```python
from build123d import *

# Parameters (mm, degrees)
SKETCH1_W               = 8
SKETCH1_H               = 8
BOSS_EXTRUDE1_DEPTH     = 3
CUT_EXTRUDE1_DEPTH      = 12.704699911
CUT_EXTRUDE1_DEPTH_BACK = 12.704699911
CUT_EXTRUDE2_DEPTH      = 11
SKETCH4_R               = 1.75
CUT_EXTRUDE3_DEPTH      = 0.4
SKETCH5_W               = 8
SKETCH5_H               = 1
BOSS_EXTRUDE2_DEPTH     = 2
FILLET1_R               = 4
CUT_EXTRUDE4_DEPTH      = 0.4
CUT_EXTRUDE5_DEPTH      = 0.5


with BuildPart() as part:
    # Sketch1 → Boss-Extrude1 (new body)
    with BuildSketch(Plane(origin=(0, 0, 0), x_dir=(1, 0, 0), z_dir=(0, 1, 0))):
        with Locations((4, 4)):
            Rectangle(SKETCH1_W, SKETCH1_H)
    extrude(amount=BOSS_EXTRUDE1_DEPTH)

    # Sketch2 → Cut-Extrude1 (cut, two sides: drawn at the far end of the back side and taken through both)
    with BuildSketch(Plane.XY.offset(-CUT_EXTRUDE1_DEPTH_BACK)):
        Polygon((0, 0), (0.6, 3), (0, 3), align=None)
        Polygon((8, 0), (7.4, 3), (8, 3), align=None)
    extrude(amount=CUT_EXTRUDE1_DEPTH + CUT_EXTRUDE1_DEPTH_BACK, mode=Mode.SUBTRACT)

    # Sketch3 → Cut-Extrude2 (cut)
    with BuildSketch(Plane(origin=(0, 0, 0), x_dir=(0, 0, -1), z_dir=(1, 0, 0))):
        Polygon((0, 0), (0.6, 3), (0, 3), align=None)
        Polygon((8, 3), (7.4, 3), (8, 0), align=None)
    extrude(amount=CUT_EXTRUDE2_DEPTH, mode=Mode.SUBTRACT)

    # Sketch4 → Cut-Extrude3 (cut)
    with BuildSketch(Plane.XZ):
        with Locations(Location((4, -3.75, 0), (0, 0, 270))):
            Circle(SKETCH4_R)
    extrude(amount=-CUT_EXTRUDE3_DEPTH, mode=Mode.SUBTRACT)

    # Sketch5 → Boss-Extrude2 (add)
    with BuildSketch(Plane.XZ):
        with Locations((4, -7.5)):
            Rectangle(SKETCH5_W, SKETCH5_H)
    extrude(amount=BOSS_EXTRUDE2_DEPTH)

    # Fillet1
    # the kernel refuses this fillet: 4 mm, written as the material it takes off along each edge
    with BuildSketch(Plane(origin=(8, -2, -16.660254038), x_dir=(0, 1, 0), z_dir=(0, 0, 1)), Plane(origin=(0, -2, 1.660254038), x_dir=(0, 1, 0), z_dir=(0, 0, -1))) as fillet1_piece_1:
        with BuildLine():
            CenterArc((4, 3.464101615), FILLET1_R, 180, 60)
            Line((0, 3.464101615), (-0.08, 3.464101615))
            Line((-0.08, 3.464101615), (-0.08, 0))
            Line((-0.08, 0), (0, -0.08))
            ThreePointArc((0, -0.08), (1, -0.08), (1.96, -0.069282032))
            Line((1.96, -0.069282032), (2, 0))
        make_face()
    extrude(amount=18.320508076, mode=Mode.SUBTRACT)

    # Sketch6 → Cut-Extrude4 (cut)
    with BuildSketch(Plane(origin=(0, 3, 0), x_dir=(1, 0, 0), z_dir=(0, 1, 0))):
        Polygon((3.623842243, 2.056832464), (3.623842243, 3.740326053), (2.162303782, 6.056832464), (3.062143525, 6.056832464), (4.007656346, 4.408595284), (4.95477173, 6.056832464), (5.854611474, 6.056832464), (4.393073013, 3.734717079), (4.393073013, 2.056832464), align=None)
    extrude(amount=-CUT_EXTRUDE4_DEPTH, mode=Mode.SUBTRACT)

    # Sketch7 → Cut-Extrude5 (cut)
    with BuildSketch(Plane(origin=(0, 3, 0), x_dir=(1, 0, 0), z_dir=(0, 1, 0))):
        with BuildLine():
            Line((6.99657775, 2.307478491), (6.650423904, 2.269617914))
            add(Edge.make_bspline(
                [(6.650423904, 2.269617914), (6.648104786, 2.286290214), (6.643740629, 2.317664439), (6.630814222, 2.360960848), (6.6128192, 2.397384178), (6.589720846, 2.426985356), (6.562208273, 2.449767653), (6.53085918, 2.465955864), (6.495693494, 2.475565581), (6.471038508, 2.476713937), (6.458236404, 2.477310221)],
                knots=[0, 0, 0, 0, 1.280716388, 2.410074291, 3.425374506, 4.35753932, 5.248331359, 6.12451615, 7.026154803, 8, 8, 8, 8], degree=3))
            add(Edge.make_bspline(
                [(6.458236404, 2.477310221), (6.449554942, 2.477097941), (6.432279271, 2.476675513), (6.407115159, 2.471312362), (6.382853927, 2.463353411), (6.359693582, 2.452081234), (6.337518567, 2.437536581), (6.316665994, 2.419545601), (6.296177185, 2.39905664), (6.277258092, 2.37431526), (6.259107425, 2.34501973), (6.243478966, 2.309156475), (6.229549311, 2.266758815), (6.217622545, 2.217619097), (6.206799126, 2.162049229), (6.197926997, 2.099824257), (6.190827571, 2.030888275), (6.1874217, 1.982610246), (6.18564025, 1.957358298)],
                knots=[0, 0, 0, 0, 0.642458078, 1.278459126, 1.898279436, 2.531842133, 3.181731979, 3.858193002, 4.57010051, 5.325711302, 6.161524323, 7.118599443, 8.217371811, 9.466325973, 10.864147948, 12.412648259, 14.123626419, 16, 16, 16, 16], degree=3))
            add(Edge.make_bspline(
                [(6.18564025, 1.957358298), (6.196703374, 1.969374309), (6.218396997, 1.992936442), (6.254393564, 2.023656049), (6.292105324, 2.049919261), (6.331942634, 2.071465901), (6.374122941, 2.087500286), (6.417882183, 2.099674887), (6.463793169, 2.1064945), (6.494994081, 2.107544715), (6.510880634, 2.108079452)],
                knots=[0, 0, 0, 0, 1.057745406, 2.074127497, 3.059409796, 4.031705469, 5.000875988, 5.977809597, 6.970362319, 8, 8, 8, 8], degree=3))
            add(Edge.make_bspline(
                [(6.510880634, 2.108079452), (6.528809934, 2.107563089), (6.564213931, 2.106543456), (6.616372239, 2.099391957), (6.666421561, 2.086532277), (6.714588312, 2.069136373), (6.761110551, 2.047230594), (6.805098359, 2.019501147), (6.847242227, 1.987169858), (6.886962554, 1.950231753), (6.923455982, 1.909566001), (6.95567607, 1.865643773), (6.982192143, 1.818330938), (7.00486021, 1.76868676), (7.021726117, 1.715731209), (7.033968982, 1.660226315), (7.04127711, 1.601662587), (7.042239139, 1.561706039), (7.042731596, 1.541252529)],
                knots=[0, 0, 0, 0, 0.99135015, 1.957564468, 2.903754199, 3.843479786, 4.78583385, 5.741106244, 6.712813504, 7.719198368, 8.735844933, 9.730198001, 10.724351158, 11.729813921, 12.742848014, 13.790983496, 14.86921809, 16, 16, 16, 16], degree=3))
            add(Edge.make_bspline(
                [(7.042731596, 1.541252529), (7.042231952, 1.519599685), (7.041257525, 1.477371451), (7.034085066, 1.415527203), (7.021415455, 1.357153196), (7.004106031, 1.301781092), (6.981716795, 1.249849655), (6.954594052, 1.200930916), (6.921819947, 1.155860856), (6.884881845, 1.114033218), (6.84370317, 1.076707467), (6.799818397, 1.043655074), (6.752740779, 1.016179585), (6.703166183, 0.993054256), (6.650243128, 0.9760833), (6.594904638, 0.963355935), (6.536700741, 0.955593381), (6.496962304, 0.954693712), (6.476625827, 0.954233298)],
                knots=[0, 0, 0, 0, 1.13287417, 2.209376133, 3.25169942, 4.254157582, 5.240146322, 6.205890558, 7.174579019, 8.150183866, 9.1206468, 10.07783463, 11.019441811, 11.967766696, 12.934309213, 13.921380422, 14.936249089, 16, 16, 16, 16], degree=3))
            add(Edge.make_bspline(
                [(6.476625827, 0.954233298), (6.454835686, 0.954842926), (6.411992392, 0.956041562), (6.349274568, 0.965905733), (6.289647802, 0.982594351), (6.233119501, 1.005900716), (6.179219819, 1.035216515), (6.128449255, 1.071632083), (6.080942348, 1.114800151), (6.036070744, 1.164136126), (5.995238787, 1.221123075), (5.960465944, 1.286988003), (5.930975089, 1.361009558), (5.906965213, 1.443377578), (5.888431321, 1.534085529), (5.875498792, 1.633141016), (5.86690889, 1.740380226), (5.866183985, 1.814672002), (5.865808519, 1.853151567)],
                knots=[0, 0, 0, 0, 0.852151446, 1.675481364, 2.476404467, 3.269281233, 4.062617998, 4.871616733, 5.707301388, 6.56955125, 7.476395267, 8.442009786, 9.475854496, 10.58877921, 11.794095973, 13.094195288, 14.494932947, 16, 16, 16, 16], degree=3))
            add(Edge.make_bspline(
                [(5.865808519, 1.853151567), (5.866346697, 1.892590697), (5.867386586, 1.968796599), (5.875754473, 2.078827487), (5.889046125, 2.180436336), (5.908408745, 2.273394012), (5.933175033, 2.357893394), (5.963200156, 2.434104295), (5.99923844, 2.501750812), (6.041138584, 2.560612949), (6.087240817, 2.61177964), (6.136777869, 2.655945181), (6.189560624, 2.693536639), (6.245587817, 2.724459089), (6.305319384, 2.747901225), (6.368188753, 2.764829378), (6.434301522, 2.775708833), (6.479587723, 2.776770851), (6.502587365, 2.777310221)],
                knots=[0, 0, 0, 0, 1.491699013, 2.882321987, 4.171520357, 5.365488089, 6.470299549, 7.49861535, 8.458736801, 9.361983288, 10.224742848, 11.058789056, 11.867429157, 12.671146298, 13.473202851, 14.288259215, 15.130652936, 16, 16, 16, 16], degree=3))
            add(Edge.make_bspline(
                [(6.502587365, 2.777310221), (6.518832845, 2.777017956), (6.550590682, 2.776446616), (6.597136362, 2.770379458), (6.641540508, 2.76110179), (6.683919501, 2.748259344), (6.723974963, 2.731060825), (6.761865954, 2.710109046), (6.797719857, 2.685460752), (6.831350121, 2.657274635), (6.862486078, 2.625465393), (6.890601127, 2.589961055), (6.915881459, 2.551190115), (6.938437714, 2.509184749), (6.957357529, 2.46354265), (6.973622233, 2.414622738), (6.98699882, 2.362319913), (6.993336088, 2.326037695), (6.99657775, 2.307478491)],
                knots=[0, 0, 0, 0, 1.036027791, 2.025301876, 2.989435482, 3.928225244, 4.845595412, 5.765526461, 6.686607585, 7.61747015, 8.561102691, 9.521661062, 10.50224679, 11.510949117, 12.559251378, 13.650572309, 14.798212656, 16, 16, 16, 16], degree=3))
        make_face()
        with BuildLine():
            add(Edge.make_bspline(
                [(6.211962365, 1.549185221), (6.212093793, 1.537753077), (6.212350595, 1.515415322), (6.216561681, 1.483001611), (6.222614755, 1.452614338), (6.230767911, 1.42408476), (6.242068736, 1.397844656), (6.255476173, 1.373367715), (6.271335314, 1.350875727), (6.295669246, 1.324486058), (6.329294099, 1.29676891), (6.373421783, 1.272086886), (6.420703408, 1.256744198), (6.453316703, 1.255075433), (6.469774865, 1.254233298)],
                knots=[0, 0, 0, 0, 0.93816693, 1.833124408, 2.679057427, 3.481731691, 4.264557977, 5.020023694, 5.770442996, 6.518065735, 7.962605608, 9.32780964, 10.651490302, 12, 12, 12, 12], degree=3))
            add(Edge.make_bspline(
                [(6.469774865, 1.254233298), (6.485365796, 1.254933043), (6.51571185, 1.256295021), (6.559046727, 1.268742487), (6.598409917, 1.288373431), (6.627266187, 1.311420354), (6.647387039, 1.333836313), (6.660907792, 1.353494474), (6.671913698, 1.375919542), (6.680911589, 1.400742183), (6.688159323, 1.427866383), (6.693107691, 1.457564676), (6.69591447, 1.48975573), (6.696351403, 1.512040132), (6.69657775, 1.52358426)],
                knots=[0, 0, 0, 0, 1.399678333, 2.724321989, 4.020062797, 5.33532049, 6.016755754, 6.724441967, 7.473839083, 8.257094862, 9.096253071, 9.995581596, 10.961638663, 12, 12, 12, 12], degree=3))
            add(Edge.make_bspline(
                [(6.69657775, 1.52358426), (6.696384678, 1.535490976), (6.696011412, 1.558510238), (6.692745041, 1.591780733), (6.687401372, 1.622537963), (6.679930507, 1.650999261), (6.669817892, 1.676783929), (6.657887501, 1.700412041), (6.643402955, 1.721242874), (6.621876525, 1.745742616), (6.590576263, 1.770429427), (6.548753213, 1.792915191), (6.501874013, 1.805662518), (6.469248141, 1.807258544), (6.452467173, 1.808079452)],
                knots=[0, 0, 0, 0, 1.008384627, 1.949510571, 2.828269698, 3.650667555, 4.437180943, 5.170285793, 5.887596972, 6.580056709, 7.926803404, 9.238379296, 10.579573008, 12, 12, 12, 12], degree=3))
            add(Edge.make_bspline(
                [(6.452467173, 1.808079452), (6.436151813, 1.807414866), (6.404464825, 1.806124136), (6.358926875, 1.793162443), (6.31725918, 1.772538153), (6.286568407, 1.748308757), (6.264936989, 1.725473324), (6.25076935, 1.706030549), (6.238437114, 1.684862342), (6.228698053, 1.661421349), (6.221189386, 1.636147459), (6.215803903, 1.608867965), (6.212544961, 1.579673333), (6.212160051, 1.559530412), (6.211962365, 1.549185221)],
                knots=[0, 0, 0, 0, 1.469034193, 2.853094746, 4.235454457, 5.641396914, 6.354997179, 7.06867986, 7.807229614, 8.560602297, 9.353235934, 10.182779392, 11.06669468, 12, 12, 12, 12], degree=3))
        make_face(mode=Mode.SUBTRACT)
    extrude(amount=-CUT_EXTRUDE5_DEPTH, mode=Mode.SUBTRACT)


solid = part.part
```
Model file for the job. Use its own axes, mm. A direction names the side the tool comes from. Round coordinates to 2 decimals unless told otherwise and drop trailing zeros. Loops run counter-clockwise (first coordinate to the right, second up) from the corner with the lowest first, then second, coordinate; pieces in that order, holes last. Notation, with made-up numbers: M -35,24 L -29,24 A22 ccw -29,57 Z; hole C 10,72.25 d8. An arc over 180 degrees is marked long. Put each result on its own line as item: value. Start each with the question number.
Item 1: Cut at C-C (x = 3.75). List the corners of the cut face in (y, z), then the cut area to 3 significant figures.
Item 2: Drop flat-ended pins along their axis: P1, Ø1, axis at y = 1.5, z = -2, coming from the +X side; P2, Ø3, axis at x = 4, z = -3.75, coming from the -Y side; P3, Ø3, axis at x = 3.5, y = 2.5, coming from the -Z side. Give the stop position or say it passes through.
Item 3: Mould opens along X. For faces 1 (the face through (1.49, -1.48, -7.49)), 2 (the face through (4.475, 2.803, -5.221)), 3 (the face through (7.7, 1.5, -4.1)) say: released by +X, released by -X, zero draft, split by the parting line, or undercut.
Item 4: Cut at A-A (z = -7.5). List the corners of the cut face in (x, y), then the cut area to 3 significant figures.
Item 5: Cut at D-D (x = 7.75). List the corners of the cut face in (y, z), then the cut area to 3 significant figures.
Item 6: Cut at B-B (y = 1.15). List the corners of the cut face in (x, z).
Item 7: Drill centre lines: line 1 along Y through (x, z) = (6.25, -6); line 2 along X through (y, z) = (0.2, -3.75); line 3 along Z through (x, y) = (3.5, -1.2). Where is each one in solid material? Low to high.
Item 8: 3-axis set-ups, long thin cutter, end or side, ignore diameter. For faces 4 (the face through (4, 0.4, -4)), 5 (the face through (3.9, 1.5, -0.3)), 6 (the face through (4.3, 2.6, -4.5)), 7 (the face through (3, 0, -2)): which of +Z, -Z, +X, -X, +Y, -Y reach the whole face in a straight line?
Answer block:
1. outline: M -2,-8 L 0,-8 L 3,-7.4 L 3,-4.86 L 2.6,-4.86 L 2.6,-2.06 L 3,-2.06 L 3,-0.6 L 0,0 L 0,-2.02 L 0.4,-2.02 L 0.4,-5.48 L 0,-5.48 L 0,-7 L -2,-7 Z
1. area: 21.7 mm2
2. P1: x = 7.8
2. P2: y = 0.4
2. P3: z = -7.8
3. face 1: released by -X
3. face 2: undercut
3. face 3: released by +X
4. outline: M 0,0 A4 ccw 3.46,-2 L 4.54,-2 A4 ccw 8,0 L 7.5,2.5 L 0.5,2.5 Z
4. area: 30.7 mm2
5. outline: M -0.38,-8 L 0,-8 L 1.25,-7.75 L 1.25,-0.25 L 0,0 L 0,-7 L -0.38,-7 Z
5. area: 10.1 mm2
6. outline: M 0.23,-7.77 L 7.77,-7.77 L 7.77,-0.23 L 0.23,-0.23 Z
7. line 1: 0 to 3
7. line 2: 0.04 to 2.25, 5.75 to 7.96
7. line 3: -8 to -7
8. face 4: -Y
8. face 5: +Z, +X, -X, +Y
8. face 6: +Y
8. face 7: +Z, +X, -X, -Y
